```python
from build123d import *

# Parameters (mm, degrees)
SKETCH1_W           = 100
SKETCH1_H           = 105
BOSS_EXTRUDE1_DEPTH = 50
FILLET1_R           = 5
SKETCH8_W           = 22.5
SKETCH8_H           = 12.5
CUT_EXTRUDE4_DEPTH  = 30
SKETCH9_W           = 33.5
SKETCH9_H           = 12.5
CUT_EXTRUDE5_DEPTH  = 12


with BuildPart() as part:
    # Sketch1 → Boss-Extrude1 (new body)
    with BuildSketch(Plane(origin=(0, 0, 0), x_dir=(1, 0, 0), z_dir=(0, 1, 0))):
        Rectangle(SKETCH1_W, SKETCH1_H)
    extrude(amount=BOSS_EXTRUDE1_DEPTH)

    # Sketch5 → Cut-Revolve1 (revolve, cut)
    with BuildSketch(Plane(origin=(0, 0, 0), x_dir=(0, 0, -1), z_dir=(1, 0, 0))):
        Polygon((-48, 50), (-15, 0), (0, 0), (0, 50), align=None)
    revolve(axis=Axis((0, -20.231136995, 0), (0, 1, 0)), mode=Mode.SUBTRACT)

    # Fillet1
    # the kernel refuses this fillet: 5 mm, written as the material it takes off along each edge
    with BuildSketch(Plane(origin=(0, 50, 0), x_dir=(0, 0, 1), z_dir=(-1, 0, 0))) as fillet1_piece_1:
        with BuildLine():
            CenterArc((48 + FILLET1_R * 0.53816526406, -FILLET1_R), FILLET1_R, 90, 56.575188817)
            Line((48 - FILLET1_R * 0.296444142502, -FILLET1_R * 0.449157791669), (48, 0))
            Line((48, 0), (48 + FILLET1_R * 0.53816526406, 0))
        make_face()
    revolve(axis=Axis((0, 50, 0), (0, 1, 0)), mode=Mode.SUBTRACT)

    # Sketch8 → Cut-Extrude4 (cut)
    with BuildSketch(Plane.XZ):
        with Locations((-6.05, 42.323299426)):
            Rectangle(SKETCH8_W, SKETCH8_H)
    extrude(amount=-CUT_EXTRUDE4_DEPTH, mode=Mode.SUBTRACT)

    # Sketch9 → Cut-Extrude5 (cut)
    with BuildSketch(Plane.XZ):
        with Locations((-6.05, 42.323299426)):
            Rectangle(SKETCH9_W, SKETCH9_H)
    extrude(amount=-CUT_EXTRUDE5_DEPTH, mode=Mode.SUBTRACT)


solid = part.part
```
For this review, take the finished solid that the model builds, in its own axes (mm). A direction names the side the tool comes from. Round coordinates to 2 decimals unless told otherwise and drop trailing zeros. Order: outer loops, then holes, each group sorted by start corner. A loop starts at its lowest first (then second) coordinate and runs counter-clockwise, first axis right, second up.
Q1. Wall thickness on line 1 (Z direction, x = -7, y = 3.5); line 2 (Z direction, x = -13.5, y = 10); line 3 (X direction, y = 6, z = 43): over which ranges is each line inside the solid? List them lowest first.
Findings below:
line 1: z = -52.5 to -15.83, 15.83 to 36.07, 48.57 to 52.5
line 2: z = -52.5 to -16.86, 16.86 to 36.07, 48.57 to 52.5
line 3: x = -50 to -22.8, 10.7 to 50
Q2. Insertion check: P1, Ø12, axis at x = -28.5, z = -29, coming from the +Y side; P2, Ø2, axis at x = -25, z = 11.5, coming from the +Y side. Each pin has a flat end and moves straight along its axis. Give the tip position at first contact, or say it passes through.
Findings below:
P1: stops at y = 47.96
P2: stops at y = 20.48
Q3. Mouldability with a two-part tool opening along X and no side actions: class faces 1 (the flat face through (-50, 25, 1)), 2 (the flat face through (-22.8, 6, 42)), 3 (the flat face through (-12, 0, -12)) as pulls with the +X half, pulls with the -X half, needs draft (parallel to the pull), parting line crosses it, or undercut.
Findings below:
face 1: pulls with the -X half
face 2: undercut
face 3: needs draft
Q4. We need section C-C, the plane z = 0. Give the boundary of the cut face in (x, y), plus the area to 3 significant figures.
Findings below:
outline: (-50, 0) - (-15, 0) - (-46.52, 47.75) arc R5 ccw to (-50, 49.95) - close; (15, 0) - (50, 0) - (50, 49.95) arc R5 ccw to (46.52, 47.75) - close
area: 1,850 mm2
Q5. We need section A-A, the plane x = 0. Give the boundary of the cut face in (y, z).
Findings below:
outline: (0, -52.5) - (50, -52.5) - (50, -50.69) arc R5 ccw to (47.75, -46.52) - (0, -15) - close; (0, 15) - (47.75, 46.52) arc R5 ccw to (50, 50.69) - (50, 52.5) - (0, 52.5) - (0, 48.57) - (30, 48.57) - (30, 36.07) - (0, 36.07) - close
Q6. Machinability: for faces 4 (the flat face through (0, 50, -52)), 5 (the flat face through (-6, 15, 36.073)), which of the approach directions +Z, -Z, +X, -X, +Y, -Y give a long, thin tool a straight path to every point of the face, cutting with its end or side? Answer none if there is none.
Findings below:
face 4: +Z, -Z, +X, -X, +Y
face 5: -Y
Q7. We need section D-D, the plane y = 45. Give the boundary of the cut face in (x, z), plus the area to 3 significant figures.
Findings below:
outline: (-50, -52.5) - (50, -52.5) - (50, 52.5) - (-50, 52.5) - close; hole circle Ø89.4 at (0, 0)
area: 4,220 mm2
Q8. We need section B-B, the plane y = 16.5. Give the boundary of the cut face in (x, z), plus the area to 3 significant figures.
Findings below:
outline: (-50, -52.5) - (50, -52.5) - (50, 52.5) - (-50, 52.5) - close; hole circle Ø51.78 at (0, 0); hole (-17.3, 36.07) - (5.2, 36.07) - (5.2, 48.57) - (-17.3, 48.57) - close
area: 8,110 mm2
